The figure shows three views and two pictorial views of one solid part (mm, origin at its lowest corner). Answer the questions. Coordinates: 2 decimals unless noted, no trailing zeros. Order: outer loops, then holes, each group sorted by start corner. A loop starts at its lowest first (then second) coordinate and runs counter-clockwise, first axis right, second up.
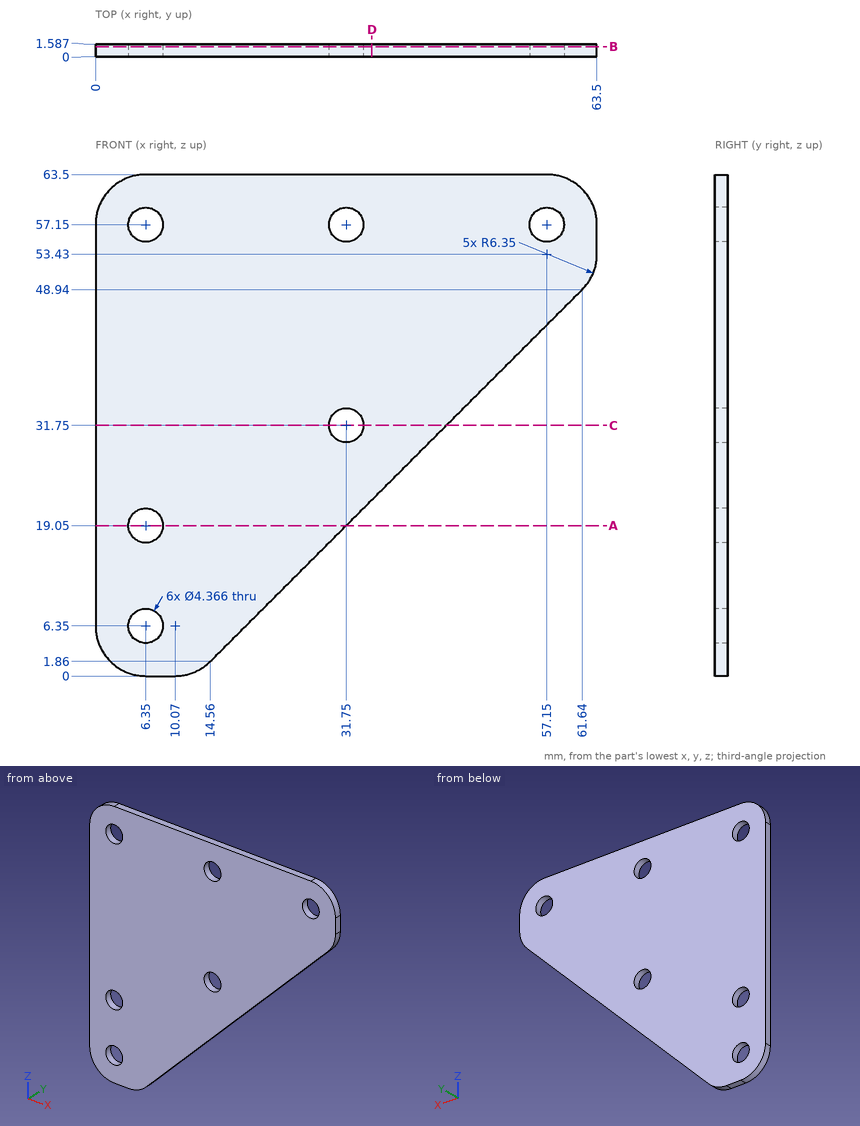
1) A cutting plane is placed at B-B, the plane y = 1.25. Count the separate pieces of the cut face and the enclosed holes in it, plus the area to 3 significant figures.
2) A cutting plane is placed at D-D, the plane x = 35. Write down the section's boundary in (y, z).
3) Straight lines are drawn through the part: probe 1 along X at (y, z) = (1.15, 57.15); probe 2 along Z at (x, y) = (5.5, 0.5); probe 3 along X at (y, z) = (0.15, 8). For each, find the intervals that lie inside material, in ascending order.
4) A cutting plane is placed at A-A, the plane z = 19.05. Write down the section's boundary in (x, y).
5) This flat-tipped pin is pushed along its axis until it touches: P1, Ø5.5, axis at x = 57.15, z = 57.15, coming from the -Y side. Where does it stop, or does it pass through?
6) A cutting plane is placed at C-C, the plane z = 31.75. Write down the section's boundary in (x, y).
Working result:
1. separate pieces: 1
1. enclosed holes: 6
1. area: 2,620 mm2
2. outline: (0, 22.3) - (1.59, 22.3) - (1.59, 63.5) - (0, 63.5) - close
3. probe 1: x = 0 to 4.17, 8.53 to 29.57, 33.93 to 54.97, 59.33 to 63.5
3. probe 2: z = 0.06 to 4.34, 8.36 to 17.04, 21.06 to 55.14, 59.16 to 63.44
3. probe 3: x = 0 to 4.92, 7.78 to 20.7
4. outline: (0, 0) - (4.17, 0) - (4.17, 1.59) - (0, 1.59) - close; (8.53, 0) - (31.75, 0) - (31.75, 1.59) - (8.53, 1.59) - close
5. P1: stops at y = 0
6. outline: (0, 0) - (29.57, 0) - (29.57, 1.59) - (0, 1.59) - close; (33.93, 0) - (44.45, 0) - (44.45, 1.59) - (33.93, 1.59) - close
